from build123d import *

# Parameters (mm, degrees)
F1_DEPTH  = 2
F2_W      = 104
F2_H      = 66
F2_W_2    = 49
F2_H_2    = 30
F3_DEPTH  = 100
F4_W      = 15
F4_H      = 2
F5_DEPTH  = 15
F7_DEPTH  = 2
F8_R      = 7.49999
F9_W      = 104
F9_H      = 66
F10_DEPTH = 2


# Not quite as in the source:
# - a fillet or chamfer is up to 0.001 mm smaller than in the source, because OpenCascade refuses the exact size


with BuildPart() as f1:
    # F0 (on Top) → F1 (new body)
    with BuildSketch(Plane.XY):
        Polygon((104, 0), (0, 0), (0, -34), (0, -66), (104, -66), (104, -34), align=None)
    extrude(amount=F1_DEPTH)

    # F2 (on face) → F3 (join)
    with BuildSketch(Plane.XY.offset(2)):
        with Locations((52, -33)):
            Rectangle(F2_W, F2_H)
        with Locations((26.5, -49)):
            Rectangle(F2_W_2, F2_H_2, mode=Mode.SUBTRACT)
        with Locations((77.5, -49)):
            Rectangle(F2_W_2, F2_H_2, mode=Mode.SUBTRACT)
        with Locations((26.5, -17)):
            Rectangle(F2_W_2, F2_H_2, mode=Mode.SUBTRACT)
        with Locations((77.5, -17)):
            Rectangle(F2_W_2, F2_H_2, mode=Mode.SUBTRACT)
    extrude(amount=F3_DEPTH)

    # F4 (on face) → F5 (join)
    with BuildSketch(Plane.XY.offset(102)):
        with Locations((27.5, -1)):
            Rectangle(F4_W, F4_H)
        with Locations((76.5, -1)):
            Rectangle(F4_W, F4_H)
    extrude(amount=F5_DEPTH)

    # F6 (on face) → F7 (cut, through all)
    with BuildSketch(Plane.XZ.offset(2)):
        with BuildLine():
            Line((79.8888604279, 107.875), (78.4364916731, 113.5))
            ThreePointArc((78.4364916731, 113.5), (76.5, 115), (74.5635083269, 113.5))
            Line((74.5635083269, 113.5), (73.1111395721, 107.875))
            ThreePointArc((73.1111395721, 107.875), (76.5, 103.5), (79.8888604279, 107.875))
        make_face()
        with BuildLine():
            Line((30.8888604279, 107.875), (29.4364916731, 113.5))
            ThreePointArc((29.4364916731, 113.5), (27.5, 115), (25.5635083269, 113.5))
            Line((25.5635083269, 113.5), (24.1111395721, 107.875))
            ThreePointArc((24.1111395721, 107.875), (27.5, 103.5), (30.8888604279, 107.875))
        make_face()
    extrude(amount=-F7_DEPTH, mode=Mode.SUBTRACT)

    # F8 (radius 7.5 in the source; OpenCascade refuses exactly that, so slightly less here)
    f8_edges = [f1.edges().sort_by_distance(p)[0] for p in [
        (84, -1, 102),
        (84, -1, 117),
        (69, -1, 117),
        (69, -1, 102),
        (35, -1, 102),
        (35, -1, 117),
        (20, -1, 117),
        (20, -1, 102),
    ]]
    fillet(f8_edges, radius=F8_R)

    # F9 (on face) → F10 (cut)
    with BuildSketch(Plane(origin=(0, 0, 0), x_dir=(1, 0, 0), z_dir=(0, 0, -1))):
        with Locations((52, 33)):
            Rectangle(F9_W, F9_H)
    extrude(amount=-F10_DEPTH, mode=Mode.SUBTRACT)


solid = f1.part
Input: part model. Units: mm. Frame: model coordinates. A direction names the side the tool comes from. Coordinates: 2 decimals unless noted, no trailing zeros. Order: outer loops, then holes, each group sorted by start corner. A loop starts at its lowest first (then second) coordinate and runs counter-clockwise, first axis right, second up.
1. Access query for faces 1 (the flat face through (77, -32, 51)), 2 (the cylindrical face through (17.745, -0.986, 104.139)), 3 (the cylindrical face through (71.139, -0.986, 114.745)). Directions: +Z, -Z, +X, -X, +Y, -Y. A direction counts if a zero-diameter tool reaches every point of the face in a straight line with its end or side. Return the directions, or none.
Checked values:
face 1: +Z, -Z
face 2: +Z, -X, +Y, -Y
face 3: +Z, +Y, -Y
2. Cut plane A-A, the plane x = 17. Return loops of the section in (y, z), plus the area to 3 significant figures.
Checked values:
outline: (-66, 2) - (-64, 2) - (-64, 102) - (-66, 102) - close; (-34, 2) - (-32, 2) - (-32, 102) - (-34, 102) - close; (-2, 2) - (0, 2) - (0, 103.5) - (-2, 103.5) - close
area: 603 mm2
3. Ray query, line 1 along Y through (x, z) = (29.5, 98); line 2 along X through (y, z) = (-23.5, 28); line 3 along X through (y, z) = (-1, 107). Return the intervals inside material, ascending.
Checked values:
line 1: y = -66 to -64, -34 to -32, -2 to 0
line 2: x = 0 to 2, 51 to 53, 102 to 104
line 3: x = 19.57 to 24, 31 to 35.43, 68.57 to 73, 80 to 84.43
4. Cut plane C-C, the plane z = 94.5. Return loops of the section in (x, y).
Checked values:
outline: (0, -66) - (104, -66) - (104, 0) - (0, 0) - close; hole (2, -64) - (51, -64) - (51, -34) - (2, -34) - close; hole (2, -32) - (51, -32) - (51, -2) - (2, -2) - close; hole (53, -64) - (102, -64) - (102, -34) - (53, -34) - close; hole (53, -32) - (102, -32) - (102, -2) - (53, -2) - close
5. Draft query along Y for faces 4 (the flat face through (26, -2, 59)), 5 (the flat face through (51, -66, 51)), 6 (the cylindrical face through (27.4, -1, 103.5)). Return one class per face: +Y half, -Y half, draft (parallel to the pull), parting line (faces both ways), or undercut.
Checked values:
face 4: undercut
face 5: -Y half
face 6: draft
6. Contact query for flat-ended pins moving along their axis: P1, Ø15, axis at y = -50.5, z = 77, coming from the -X side; P2, Ø5.5, axis at x = 27.5, z = 107, coming from the -Y side; P3, Ø3, axis at x = 72.5, z = 104.5, coming from the -Y side. Output: stop coordinate, or through.
Checked values:
P1: stops at x = 0
P2: passes through
P3: stops at y = -2
7. Cut plane B-B, the plane y = -14. Return loops of the section in (x, z).
Checked values:
outline: (0, 2) - (2, 2) - (2, 102) - (0, 102) - close; (51, 2) - (53, 2) - (53, 102) - (51, 102) - close; (102, 2) - (104, 2) - (104, 102) - (102, 102) - close
